```python
from build123d import *

# Parameters (mm, degrees)
SKETCH_1_R      = 5.05
SKETCH_1_R_2    = 2.05
SKETCH_1_W      = 8.1
SKETCH_1_H      = 2.1
EXTRUDE_1_DEPTH = 2


with BuildPart() as part:
    # 草图1 → 凸台-拉伸1 (new body)
    with BuildSketch(Plane.XY):
        with BuildLine():
            ThreePointArc((-7.35497191, -38.809204942), (0, 39.5), (7.35497191, -38.809204942))
            ThreePointArc((7.35497191, -38.809204942), (0, -27.662081143), (-7.35497191, -38.809204942))
        make_face()
        Circle(SKETCH_1_R, mode=Mode.SUBTRACT)
        with Locations((-17.67766953, -17.67766953)):
            Circle(SKETCH_1_R_2, mode=Mode.SUBTRACT)
        with Locations((-17.67766953, 17.67766953)):
            Circle(SKETCH_1_R_2, mode=Mode.SUBTRACT)
        with Locations((17.67766953, 17.67766953)):
            Circle(SKETCH_1_R_2, mode=Mode.SUBTRACT)
        with Locations((17.67766953, -17.67766953)):
            Circle(SKETCH_1_R_2, mode=Mode.SUBTRACT)
        with Locations((31, 10.05)):
            Circle(SKETCH_1_R_2, mode=Mode.SUBTRACT)
        with Locations(Location((31, -10.05, 0), (0, 0, 180))):
            Circle(SKETCH_1_R_2, mode=Mode.SUBTRACT)
        with Locations((-31, -10.05)):
            Circle(SKETCH_1_R_2, mode=Mode.SUBTRACT)
        with Locations(Location((-31, 10.05, 0), (0, 0, 180))):
            Circle(SKETCH_1_R_2, mode=Mode.SUBTRACT)
        with Locations((-14.05, 0)):
            Circle(SKETCH_1_R_2, mode=Mode.SUBTRACT)
        with Locations(Location((14.05, 0, 0), (0, 0, 180))):
            Circle(SKETCH_1_R_2, mode=Mode.SUBTRACT)
        with Locations((16, -10.05)):
            Rectangle(SKETCH_1_W, SKETCH_1_H, mode=Mode.SUBTRACT)
        with Locations((16, 10.05)):
            Rectangle(SKETCH_1_W, SKETCH_1_H, mode=Mode.SUBTRACT)
        with Locations((-16, 10.05)):
            Rectangle(SKETCH_1_W, SKETCH_1_H, mode=Mode.SUBTRACT)
        with Locations((-16, -10.05)):
            Rectangle(SKETCH_1_W, SKETCH_1_H, mode=Mode.SUBTRACT)
    extrude(amount=EXTRUDE_1_DEPTH)


solid = part.part
```
Geometry: final body of the model. Coordinates: model frame, mm. Round coordinates to 2 decimals unless told otherwise and drop trailing zeros. Write each loop counter-clockwise with the first axis right and the second up, starting at its lowest first coordinate (ties: lowest second). Pieces come first, ordered by that corner, then holes. Notation, with made-up numbers: M 86.25,-2 L 95.25,-2 A5 ccw 95.25,3 Z; hole C 20.5,-21 d10. An arc over 180 degrees is marked long. Answer in a Markdown table with one row per item. Add a question column.
(1) Ray query, L1, parallel to X at y = -17, z = 0.55; L2, parallel to X at y = 0.5, z = 0.1; L3, parallel to X at y = 9.5, z = 0.9. Return the intervals inside material, ascending.
(2) Cut plane B-B, the plane x = 0. Return the cut outline in (y, z), then the cut area to 3 significant figures.
(3) Cut plane C-C, the plane y = -10.05. Return the cut outline in (x, z).
(4) Draft query along Y for faces 1 (the face through (11.95, 10, 1)), 2 (the face through (1, -8, 0)), 3 (the face through (-11.95, -10, 1)), 4 (the face through (-1.633, 39.466, 0.986)). Return one class per face: pulls with the +Y half, pulls with the -Y half, needs draft (parallel to the pull), parting line crosses it, or undercut.
(5) Contact query for flat-ended pins moving along their axis: pin 1 (1 mm diameter, centred on x = 16, z = 1, fed in from -Y); pin 2 (0.6 mm diameter, centred on y = 10, z = 1.5, fed in from -X); pin 3 (1 mm diameter, centred on x = 17, z = 1.5, fed in from +Y). Output: stop coordinate, or through.
(6) Cut plane D-D, the plane x = -30.5. Return the cut outline in (y, z), then the cut area to 3 significant figures.
(7) Cut plane A-A, the plane y = 0. Return the cut outline in (x, z), then the cut area to 3 significant figures.
Established:
| question | item | result |
|---|---|---|
| 1 | L1 | -35.65 to -19.61, -15.74 to 15.74, 19.61 to 35.65 |
| 1 | L2 | -39.5 to -16.04, -12.06 to -5.03, 5.03 to 12.06, 16.04 to 39.5 |
| 1 | L3 | -38.34 to -32.97, -29.03 to -20.05, -11.95 to 11.95, 20.05 to 29.03, 32.97 to 38.34 |
| 2 | outline | M -27.66,0 L -5.05,0 L -5.05,2 L -27.66,2 Z; M 5.05,0 L 39.5,0 L 39.5,2 L 5.05,2 Z |
| 2 | area | 114 mm² |
| 3 | outline | M -38.2,0 L -33.05,0 L -33.05,2 L -38.2,2 Z; M -28.95,0 L -20.05,0 L -20.05,2 L -28.95,2 Z; M -11.95,0 L 11.95,0 L 11.95,2 L -11.95,2 Z; M 20.05,0 L 28.95,0 L 28.95,2 L 20.05,2 Z; M 33.05,0 L 38.2,0 L 38.2,2 L 33.05,2 Z |
| 4 | face 1 | undercut |
| 4 | face 2 | needs draft |
| 4 | face 3 | undercut |
| 4 | face 4 | parting line crosses it |
| 5 | pin 1 | y = -36.33 |
| 5 | pin 2 | x = -38.29 |
| 5 | pin 3 | y = 35.89 |
| 6 | outline | M -25.1,0 L -12.04,0 L -12.04,2 L -25.1,2 Z; M -8.06,0 L 8.06,0 L 8.06,2 L -8.06,2 Z; M 12.04,0 L 25.1,0 L 25.1,2 L 12.04,2 Z |
| 6 | area | 84.5 mm² |
| 7 | outline | M -39.5,0 L -16.1,0 L -16.1,2 L -39.5,2 Z; M -12,0 L -5.05,0 L -5.05,2 L -12,2 Z; M 5.05,0 L 12,0 L 12,2 L 5.05,2 Z; M 16.1,0 L 39.5,0 L 39.5,2 L 16.1,2 Z |
| 7 | area | 121 mm² |
